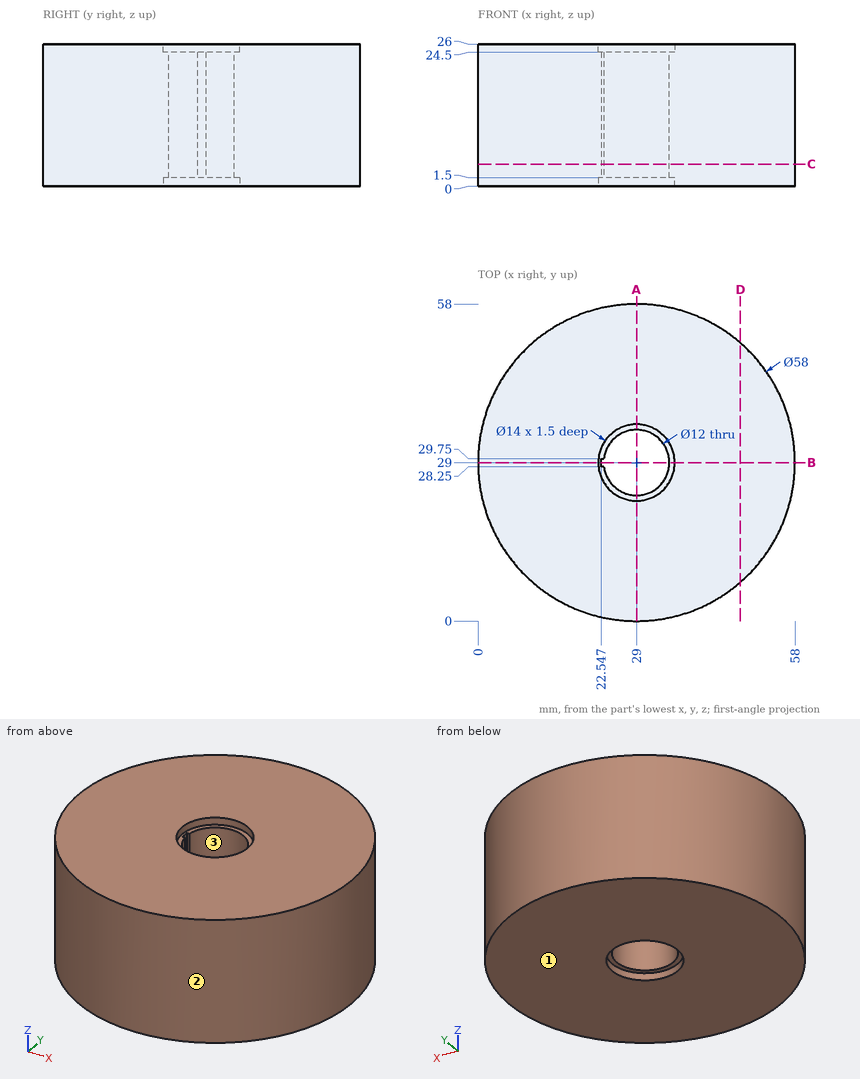
Input: dimensioned drawing with shaded views. Units: mm. Origin: part minimum x, y, z. Give positions to 0.01 mm unless a question says otherwise; leave off trailing zeros. Loops run counter-clockwise (first coordinate to the right, second up) from the corner with the lowest first, then second, coordinate; pieces in that order, holes last. Notation, with made-up numbers: M 76.25,-35 L 122.25,-35 A10 ccw 122.25,-19 Z; hole C 46,8.25 d11. An arc over 180 degrees is marked long. Put each result on its own line as item: value. Start each with the question number.
1) Cut plane A-A (x = 29). Output: boundary loops of the cut face in (y, z), then the cut area to 3 significant figures.
2) Pull-direction query (X, two-part tool) for the marked faces 1, 2 and 3; classes: pulls with the +X half, pulls with the -X half, needs draft (parallel to the pull), parting line crosses it, or undercut.
3) Cut plane C-C (z = 4). Output: boundary loops of the cut face in (x, y).
4) Contact query for flat-ended pins moving along their axis: pin 1 (3 mm diameter, centred on x = 15.5, z = 13, fed in from -Y); pin 2 (9.5 mm diameter, centred on x = 29, y = 29, fed in from +Z); pin 3 (1.5 mm diameter, centred on y = 25, z = 5.5, fed in from -X); pin 4 (8 mm diameter, centred on y = 51, z = 17.5, fed in from -X). Output: stop coordinate, or through.
5) Cut plane D-D (x = 48). Output: boundary loops of the cut face in (y, z), then the cut area to 3 significant figures.
6) Ray query, line 1 along Y through (x, z) = (29, 0.3); line 2 along Y through (x, z) = (29, 13.75); line 3 along X through (y, z) = (23.5, 20.25). Return the intervals inside material, ascending.
7) Cut plane B-B (y = 29). Output: boundary loops of the cut face in (x, z).
Verdict:
1. outline: M 0,0 L 22,0 L 22,1.5 L 23,1.5 L 23,24.5 L 22,24.5 L 22,26 L 0,26 Z; M 35,1.5 L 36,1.5 L 36,0 L 58,0 L 58,26 L 36,26 L 36,24.5 L 35,24.5 Z
1. area: 1,190 mm2
2. face 1: needs draft
2. face 2: parting line crosses it
2. face 3: undercut
3. outline: C 29,29 d58; hole M 22.55,28.25 L 23.05,28.25 A6 ccw long 23.05,29.75 L 22.55,29.75 Z
4. pin 1: y = 2.6
4. pin 2: through
4. pin 3: x = 0.18
4. pin 4: x = 6.26
5. outline: M 7.09,0 L 50.91,0 L 50.91,26 L 7.09,26 Z
5. area: 1,140 mm2
6. line 1: 0 to 22, 36 to 58
6. line 2: 0 to 23, 35 to 58
6. line 3: 0.53 to 26.6, 31.4 to 57.47
7. outline: M 0,0 L 22,0 L 22,1.5 L 22.55,1.5 L 22.55,24.5 L 22,24.5 L 22,26 L 0,26 Z; M 35,1.5 L 36,1.5 L 36,0 L 58,0 L 58,26 L 36,26 L 36,24.5 L 35,24.5 Z
